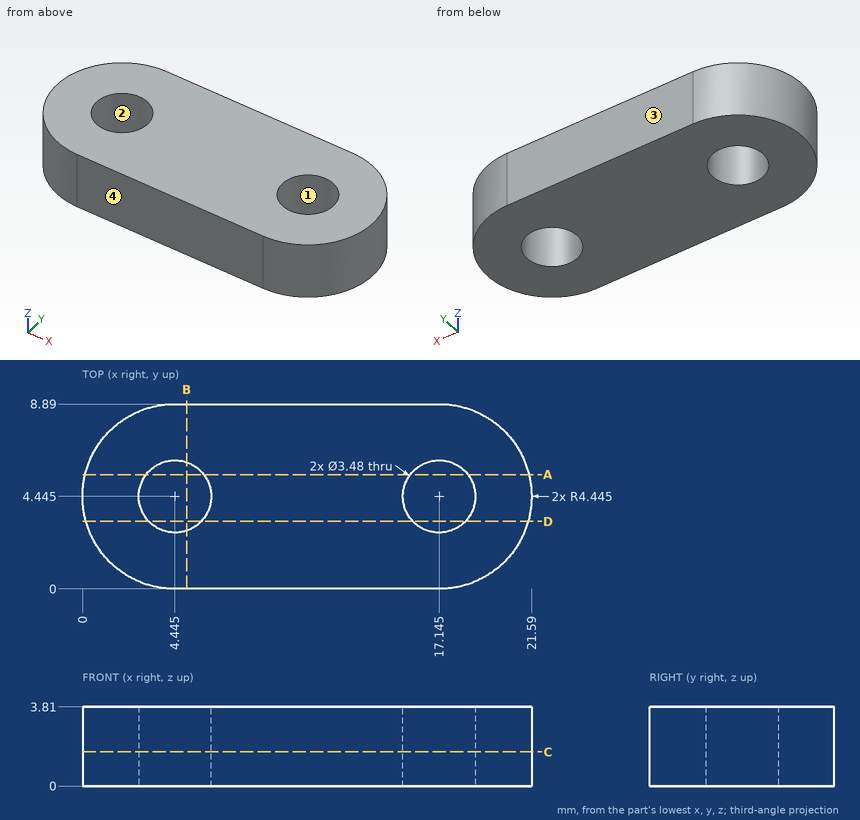
Here's the drawing with two shaded views (mm, measured from the low corner). I have some questions. Give positions to 0.01 mm unless a question says otherwise; leave off trailing zeros. Loops run counter-clockwise (first coordinate to the right, second up) from the corner with the lowest first, then second, coordinate; pieces in that order, holes last. Notation, with made-up numbers: (-7.5, -37) - (38.5, -37) arc R23 ccw to (38.5, 2) - close; hole circle Ø5 at (44.25, -22.5). An arc over 180 degrees is marked (long way). Answer in a Markdown table with one row per item. Add a question column.
Q1. For pin 1 (2 mm diameter, centred on y = 2.5, z = 0.5, fed in from +X); pin 2 (4.5 mm diameter, centred on x = 4.445, y = 4.445, fed in from +Z), each with a flat end and sliding along its axis, tell me the tip position at first contact or that it passes through.
Q2. If we section it at D-D (y = 3.25): List the corners of the cut face in (x, z) for me.
Q3. If we section it at B-B (x = 5): List the corners of the cut face in (y, z) for me, plus the area to 3 significant figures.
Q4. If we section it at A-A (y = 5.5): List the corners of the cut face in (x, z) for me.
Q5. Please list where these lines run through material, in increasing order: L1, parallel to X at y = 4.5, z = 2; L2, parallel to X at y = 5.5, z = 2.9; L3, parallel to Y at x = 4.75, z = 2.85. Write a range as from..to.
Q6. We'd pull the mould along Y, two halves only. Please class the marked faces 1, 2, 3 and 4: +Y half, -Y half, draft (parallel to the pull), parting line (faces both ways), or undercut.
Q7. If we section it at C-C (z = 1.65): List the corners of the cut face in (x, y) for me (1 decimal), plus the area to 3 significant figures.
The answers:
| question | item | result |
|---|---|---|
| 1 | pin 1 | stops at x = 21.49 |
| 1 | pin 2 | stops at z = 3.81 |
| 2 | outline | (0.16, 0) - (3.18, 0) - (3.18, 3.81) - (0.16, 3.81) - close; (5.71, 0) - (15.88, 0) - (15.88, 3.81) - (5.71, 3.81) - close; (18.41, 0) - (21.43, 0) - (21.43, 3.81) - (18.41, 3.81) - close |
| 3 | outline | (0, 0) - (2.8, 0) - (2.8, 3.81) - (0, 3.81) - close; (6.09, 0) - (8.89, 0) - (8.89, 3.81) - (6.09, 3.81) - close |
| 3 | area | 21.3 mm^2 |
| 4 | outline | (0.13, 0) - (3.06, 0) - (3.06, 3.81) - (0.13, 3.81) - close; (5.83, 0) - (15.76, 0) - (15.76, 3.81) - (5.83, 3.81) - close; (18.53, 0) - (21.46, 0) - (21.46, 3.81) - (18.53, 3.81) - close |
| 5 | L1 | x = 0..2.71, 6.18..15.41, 18.88..21.59 |
| 5 | L2 | x = 0.13..3.06, 5.83..15.76, 18.53..21.46 |
| 5 | L3 | y = 0..2.73, 6.16..8.89 |
| 6 | face 1 | undercut |
| 6 | face 2 | undercut |
| 6 | face 3 | +Y half |
| 6 | face 4 | -Y half |
| 7 | outline | (4.4, 0) - (17.1, 0) arc R4.4 ccw to (17.1, 8.9) - (4.4, 8.9) arc R4.4 ccw to start; hole circle Ø3.5 at (4.4, 4.4); hole circle Ø3.5 at (17.1, 4.4) |
| 7 | area | 156 mm^2 |
